The model under review builds one solid part; all positions refer to its coordinate system, in mm. A direction names the side the tool comes from. Coordinates: 2 decimals unless noted, no trailing zeros. Order: outer loops, then holes, each group sorted by start corner. A loop starts at its lowest first (then second) coordinate and runs counter-clockwise, first axis right, second up. Notation, with made-up numbers: M 63,-34.75 L 82,-34.75 A29 cw 82,-5.75 Z; hole C 29.5,5.25 d3. An arc over 180 degrees is marked long. Write each question's results on one line, items separated by ' | '.
from build123d import *

# Parameters (mm, degrees)
BOSS_EXTRUDE1_DEPTH = 5
SKETCH1_3_R         = 1.1000000000006245
SKETCH1_3_R_2       = 1.1000000000006236
BOSS_EXTRUDE2_DEPTH = 7
SKETCH1_6_R         = 1.1000000000006236
SKETCH1_6_R_2       = 1.1000000000006245
CUT_EXTRUDE3_DEPTH  = 5
FILLET1_R           = 4
FILLET2_R           = 2
CUT_EXTRUDE8_START  = 4
CUT_EXTRUDE8_DEPTH  = 1


with BuildPart() as part:
    # Sketch1 → Boss-Extrude1 (new body)
    with BuildSketch(Plane.XY):
        with BuildLine():
            Line((-83.13843876330769, 48.0000000000023), (-69.28203230275663, 40.00000000000234))
            ThreePointArc((-69.28203230275663, 40.00000000000234), (-27.361611466054974, 75.17540966287518), (27.361611466052146, 75.17540966287518))
            Line((27.361611466052146, 75.17540966287518), (32.833933759262855, 90.21049159544972))
            ThreePointArc((32.833933759262855, 90.21049159544972), (-32.83393375926571, 90.21049159544971), (-83.13843876330769, 48.0000000000023))
        make_face()
    extrude(amount=BOSS_EXTRUDE1_DEPTH)

    # Sketch1<3> → Boss-Extrude2 (add)
    with BuildSketch(Plane.XY):
        with BuildLine():
            Line((-13.453363993461283, 84.94119729118435), (-12.514757203219895, 79.01506724761352))
            ThreePointArc((-12.514757203219894, 79.01506724761353), (-1.39977e-12, 80.00000000000253), (12.514757203217084, 79.01506724761356))
            Line((12.514757203217078, 79.01506724761352), (13.453363993458465, 84.94119729118435))
            Line((13.453363993458465, 84.94119729118435), (14.079101853619393, 88.89195065356492))
            Line((14.079101853619393, 88.89195065356492), (15.017708643860779, 94.81808069713574))
            ThreePointArc((15.017708643860784, 94.81808069713577), (-1.40067e-12, 96.00000000000256), (-15.017708643863598, 94.81808069713577))
            Line((-15.017708643863596, 94.81808069713574), (-14.07910185362221, 88.89195065356492))
            Line((-14.07910185362221, 88.89195065356492), (-13.453363993461283, 84.94119729118435))
        make_face()
        with Locations(Location((-8.000000000001409, 88.00000000000252, 0), (0, 0, 180))):
            Circle(SKETCH1_3_R, mode=Mode.SUBTRACT)
        with Locations((7.999999999998591, 88.00000000000252)):
            Circle(SKETCH1_3_R_2, mode=Mode.SUBTRACT)
    extrude(amount=BOSS_EXTRUDE2_DEPTH)

    # Sketch1<6> → Cut-Extrude3 (cut)
    with BuildSketch(Plane.XY):
        with BuildLine():
            Line((-75.48035111508972, 49.01751315135477), (-72.125668843308, 46.83895701129465))
            ThreePointArc((-72.12566884330799, 46.83895701129467), (-46.83895701129383, 72.12566884330892), (-13.453363993461279, 84.94119729118435))
            Line((-13.453363993461283, 84.94119729118435), (-14.07910185362221, 88.89195065356492))
            ThreePointArc((-14.079101853622205, 88.89195065356492), (-49.01751315135395, 75.4803511150906), (-75.48035111508973, 49.01751315135477))
        make_face()
        with BuildLine():
            Line((14.079101853619393, 88.89195065356492), (13.453363993458465, 84.94119729118435))
            ThreePointArc((13.453363993458456, 84.94119729118435), (19.345790673570992, 83.79582557153273), (25.14396660615395, 82.24220901282357))
            Line((25.143966606153956, 82.24220901282357), (26.31345342504491, 86.06742803667572))
            ThreePointArc((26.31345342504492, 86.06742803667575), (20.245594890946464, 87.69330583067372), (14.079101853619395, 88.89195065356492))
        make_face()
        with Locations((7.999999999998591, 88.00000000000252)):
            Circle(SKETCH1_6_R)
        with Locations(Location((-8.000000000001409, 88.00000000000252, 0), (0, 0, 180))):
            Circle(SKETCH1_6_R_2)
    extrude(amount=CUT_EXTRUDE3_DEPTH, mode=Mode.SUBTRACT)

    # Fillet1
    fillet1_edges = [part.edges().sort_by_distance(p)[0] for p in [
        (27.361611466052143, 75.17540966287518, 2.5),
        (-69.28203230275663, 40.000000000002345, 2.5),
        (-83.1384387633077, 48.0000000000023, 2.5),
        (32.83393375926286, 90.21049159544972, 2.5),
    ]]
    fillet(fillet1_edges, radius=FILLET1_R)

    # Fillet2
    fillet2_edges = [part.edges().sort_by_distance(p)[0] for p in [
        (13.45336399345846, 84.94119729118435, 2.5),
        (14.079101853619393, 88.89195065356492, 2.5),
        (-13.45336399346129, 84.94119729118435, 2.5),
        (-14.079101853622209, 88.89195065356492, 2.5),
        (-72.125668843308, 46.83895701129467, 2.5),
        (-75.48035111508975, 49.01751315135476, 2.5),
        (26.313453425044912, 86.06742803667574, 2.5),
        (25.143966606153953, 82.24220901282357, 2.5),
    ]]
    fillet(fillet2_edges, radius=FILLET2_R - 0.0001)  # a hair under: the kernel refuses the full size

    # Sketch1<11> → Cut-Extrude8 (cut)
    with BuildSketch(Plane.XY.offset(CUT_EXTRUDE8_START)):
        with BuildLine():
            ThreePointArc((-60.90905171355247, 74.20301489398085), (-61.063509146668466, 74.07596000522229), (-61.21770154690506, 73.9485836058718))
            Line((-61.21770154690517, 73.9485836058717), (-57.40122339078805, 69.31882538850002))
            ThreePointArc((-57.40122339078971, 69.31882538849865), (-57.247039825001984, 69.44621250489581), (-57.092573557434, 69.5732566766103))
            Line((-57.09257355743297, 69.57325667661115), (-60.909051713550085, 74.20301489398283))
        make_face()
        with BuildLine():
            ThreePointArc((-67.14449326003556, 68.61207637765807), (-67.28728937278758, 68.47204311880354), (-67.42979343969591, 68.33171267193941))
            Line((-67.42979343969681, 68.33171267193853), (-63.22432811901289, 64.05220007072279))
            ThreePointArc((-63.22432811901119, 64.05220007072444), (-63.081833786988334, 64.19254042387854), (-62.939027939352314, 64.33256377644165))
            Line((-62.93902793935119, 64.33256377644273), (-67.14449326003512, 68.61207637765848))
        make_face()
        with BuildLine():
            ThreePointArc((-72.86892466985591, 62.49895853099788), (-72.9989726976045, 62.34701263970007), (-73.12870388919032, 62.19479614475513))
            Line((-73.12870388918984, 62.19479614475569), (-68.5662575343589, 58.298098834631475))
            ThreePointArc((-68.56625753435887, 58.298098834631524), (-68.43653690400481, 58.45032434971835), (-68.30647831502658, 58.60226122087179))
            Line((-68.30647831502684, 58.60226122087151), (-72.86892466985778, 62.498958530995715))
        make_face()
        with BuildLine():
            Line((16.639553027860302, 100.6343880514797), (14.331087155641026, 86.8395399557962))
            ThreePointArc((14.331087155641026, 86.8395399557962), (14.54451947105813, 86.80404778668378), (14.757863892002872, 86.76803104912538))
            Line((14.757863892002872, 86.76803104912538), (17.066344573354787, 100.56296764072263))
            Line((17.066344573354787, 100.56296764072263), (16.639553027860302, 100.6343880514797))
        make_face()
        with BuildLine():
            Line((25.73337251273005, 98.70106424012083), (22.231449806724747, 85.16013385550725))
            ThreePointArc((22.231449806724747, 85.16013385550725), (22.037877706171837, 85.21043190246515), (21.844191809986345, 85.26028995356089))
            Line((21.844191809986345, 85.26028995356089), (25.34611345657903, 98.80121624174181))
            Line((25.34611345657903, 98.80121624174181), (25.73337251273005, 98.70106424012083))
        make_face()
        with BuildLine():
            Line((42.116005821693015, 92.89966951845646), (36.3159273051723, 80.17255878891613))
            ThreePointArc((36.3159273051723, 80.17255878891613), (36.49801466794809, 80.08982884296243), (36.67991356817236, 80.00668534208985))
            Line((36.67991356817236, 80.00668534208985), (42.47999033003967, 92.733792221395))
            Line((42.47999033003967, 92.733792221395), (42.116005821693015, 92.89966951845646))
        make_face()
        with BuildLine():
            Line((-16.639553027863123, 100.6343880514797), (-14.331087155646365, 86.83953995579603))
            ThreePointArc((-14.331087155646365, 86.83953995579603), (-14.544519471062088, 86.80404778668402), (-14.757863892005375, 86.76803104912547))
            Line((-14.757863892005375, 86.76803104912547), (-17.066344573355888, 100.56296764072306))
            Line((-17.066344573355888, 100.56296764072306), (-16.639553027863123, 100.6343880514797))
        make_face()
        with BuildLine():
            Line((-25.346113456581847, 98.80121624174181), (-21.8441918099951, 85.26028995355922))
            ThreePointArc((-21.8441918099951, 85.26028995355922), (-22.03787770624786, 85.21043190244556), (-22.231449806868046, 85.16013385546994))
            Line((-22.231449806868046, 85.16013385546994), (-25.733372512730377, 98.70106424012063))
            Line((-25.733372512730377, 98.70106424012063), (-25.346113456581847, 98.80121624174181))
        make_face()
        with BuildLine():
            Line((-34.251374684060885, 96.12374945737389), (-29.568170243810847, 82.89878809264937))
            ThreePointArc((-29.568170243810847, 82.89878809264937), (-29.379717798712498, 82.96576366709935), (-29.191113647373975, 83.03231083634289))
            Line((-29.191113647373975, 83.03231083634289), (-33.87431808762401, 96.25727220106741))
            Line((-33.87431808762401, 96.25727220106741), (-34.251374684060885, 96.12374945737389))
        make_face()
        with BuildLine():
            Line((-42.47999033004247, 92.73379222139498), (-36.67991356817387, 80.00668534209034))
            ThreePointArc((-36.67991356817387, 80.00668534209034), (-36.49801466794875, 80.0898288429634), (-36.31592730517207, 80.1725587889175))
            Line((-36.31592730517207, 80.1725587889175), (-42.11600582169416, 92.89966951845659))
            Line((-42.11600582169416, 92.89966951845659), (-42.47999033004247, 92.73379222139498))
        make_face()
        with BuildLine():
            Line((-50.40062368063963, 88.67853703576704), (-43.51337750884637, 76.50537063873087))
            ThreePointArc((-43.51337750884637, 76.50537063873087), (-43.33941722242662, 76.6040512872355), (-43.16523314692608, 76.70233638011615))
            Line((-43.16523314692608, 76.70233638011615), (-50.052481402265904, 88.87550645980734))
            Line((-50.052481402265904, 88.87550645980734), (-50.40062368063963, 88.67853703576704))
        make_face()
        with BuildLine():
            Line((-57.937677852298485, 83.94838463773227), (-50.01567837258084, 72.42180386960484))
            ThreePointArc((-50.01567837258084, 72.42180386960484), (-49.850980642786205, 72.53527064642093), (-49.68602550055159, 72.64836287732517))
            Line((-49.68602550055159, 72.64836287732517), (-57.6080273768518, 84.17494713250092))
            Line((-57.6080273768518, 84.17494713250092), (-57.937677852298485, 83.94838463773227))
        make_face()
        with BuildLine():
            Line((-82.9591200723337, 59.41983064866502), (-71.53733737082064, 51.27275222465001))
            ThreePointArc((-71.53733737082064, 51.27275222465001), (-71.653662958767, 51.11006107791678), (-71.769618553105, 50.94710601730748))
            Line((-71.769618553105, 50.94710601730748), (-83.19140125461807, 59.09418444132249))
            Line((-83.19140125461807, 59.09418444132249), (-82.9591200723337, 59.41983064866502))
        make_face()
    extrude(amount=CUT_EXTRUDE8_DEPTH, mode=Mode.SUBTRACT)


solid = part.part
1) Take a section at B-B on z = 2.5. Count the separate pieces of the cut face and the enclosed holes in it, plus the area to 3 significant figures.
Solutions:
separate pieces: 1 | enclosed holes: 4 | area: 1,610 mm2
2) Take a section at C-C on x = -8. State the section outline as (y, z) points.
Solutions:
outline: M 79.6,0 L 86.9,0 L 86.9,7 L 79.6,7 Z; M 89.1,0 L 95.67,0 L 95.67,7 L 89.1,7 Z
3) For pin 1 (2.5 mm diameter, centred on x = -26.5, y = 89, fed in from +Z); pin 2 (1 mm diameter, centred on y = 59.5, z = 4, fed in from -X); pin 3 (1 mm diameter, centred on x = 14.5, z = 5, fed in from -Y), all flat-tipped, find the tip position at first contact; note any pin that passes through.
Solutions:
pin 1: z = 5 | pin 2: x = -75.73 | pin 3: y = 78.58
4) For faces 4 (the flat face through (-59.2, 71.8, 4)), 5 (the cylindrical face through (26.68, 76.61, 2.54)), 6 (the cylindrical face through (19.29, 83.81, 2.46)), 7 (the flat face through (-35, 86, 5)), 8 (the flat face through (13.76, 86.88, 5.82)), list the 3-axis set-ups (+Z, -Z, +X, -X, +Y, -Y) from which the entire face can be reached by the end or side of a thin tool; tool diameter is ignored.
Solutions:
face 4: +Z | face 5: +Z, -Z, -Y | face 6: +Z, -Z | face 7: +Z, -X, +Y, -Y | face 8: +Z, +X, -Y
5) To check wall thickness, follow line 1 along X through (y, z) = (56, 2); line 2 along Z through (x, y) = (18, 82); line 3 along Y through (x, z) = (24, 1.5). State the ranges of each line that lie inside material, in increasing order.
Solutions:
line 1: -77.97 to -70.46, -65.27 to -57.13 | line 2: 0 to 5 | line 3: 76.32 to 82.73, 86.74 to 92.95
6) Take a section at A-A on x = -53. State the section outline as (y, z) points.
Solutions:
outline: M 59.92,0 L 67.73,0 L 67.73,5 L 59.92,5 Z; M 72.74,0 L 80.04,0 L 80.04,5 L 77.47,5 L 77.47,4 L 76.76,4 L 76.76,5 L 72.74,5 Z
7) The part is to be moulded in two halves that separate along X. For faces 1 (the cylindrical face through (-7.86, 86.91, 3.45)), 2 (the flat face through (30.047, 82.555, 2.465)), 3 (the flat face through (-68, 64, 5)), say which applies: pulls with the +X half, pulls with the -X half, needs draft (parallel to the pull), parting line crosses it, or undercut.
Solutions:
face 1: undercut | face 2: pulls with the +X half | face 3: needs draft
